Here's how the part is built. I have some questions about the finished solid (model axes, mm). Face numbers are marked on the shaded views. Coordinates: 2 decimals unless noted, no trailing zeros. Write each loop counter-clockwise with the first axis right and the second up, starting at its lowest first coordinate (ties: lowest second). Pieces come first, ordered by that corner, then holes. Notation, with made-up numbers: (-38, 2.25) - (0, 2.25) arc R16 cw to (0, 20.25) - close; hole circle Ø11 at (26, 71.5). An arc over 180 degrees is marked (long way). Answer in a Markdown table with one row per item. Add a question column.
Item 1: Imagine slicing it at A-A (x = 127). Please give me the cut outline in (y, z), plus the area to 3 significant figures.
Item 2: If I drill on probe 1 along Z at (x, y) = (25.4, -17.5); probe 2 along X at (y, z) = (-17.25, -70); probe 3 along X at (y, z) = (-11, -94.5), over which ranges is the centre line in solid material (lowest first)? Write a range as from..to.
Item 3: Imagine slicing it at C-C (y = -21.5). State how many separate pieces and enclosed holes the cut face has, plus the area to 3 significant figures.
Item 4: Imagine slicing it at B-B (z = -63.5). Please give me the cut outline in (x, y).
Item 5: We'd pull the mould along X, two halves only. Please class the marked faces 1, 2, 3 and 4: +X half, -X half, draft (parallel to the pull), parting line (faces both ways), or undercut.
Item 6: Imagine slicing it at D-D (z = -97.5). Please give me the cut outline in (x, y).
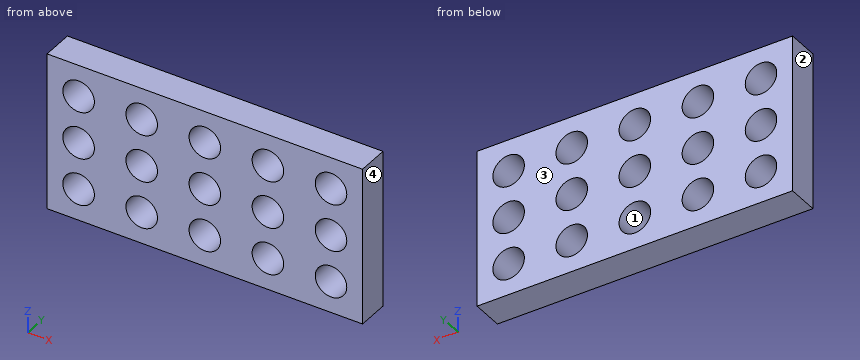
from build123d import *

# Parameters (mm, degrees)
F0_W     = 254
F0_H     = 127
F0_R     = 12.7
F1_DEPTH = 25.4


with BuildPart() as f1:
    # F0 (on Front) → F1 (new body)
    with BuildSketch(Plane.XZ):
        with Locations((127, -63.5)):
            Rectangle(F0_W, F0_H)
        with Locations((25.4, -101.6)):
            Circle(F0_R, mode=Mode.SUBTRACT)
        with Locations((76.2, -101.6)):
            Circle(F0_R, mode=Mode.SUBTRACT)
        with Locations((127, -101.6)):
            Circle(F0_R, mode=Mode.SUBTRACT)
        with Locations((177.8, -101.6)):
            Circle(F0_R, mode=Mode.SUBTRACT)
        with Locations((228.6, -101.6)):
            Circle(F0_R, mode=Mode.SUBTRACT)
        with Locations((25.4, -63.5)):
            Circle(F0_R, mode=Mode.SUBTRACT)
        with Locations((76.2, -63.5)):
            Circle(F0_R, mode=Mode.SUBTRACT)
        with Locations((25.4, -25.4)):
            Circle(F0_R, mode=Mode.SUBTRACT)
        with Locations((76.2, -25.4)):
            Circle(F0_R, mode=Mode.SUBTRACT)
        with Locations((127, -63.5)):
            Circle(F0_R, mode=Mode.SUBTRACT)
        with Locations((177.8, -63.5)):
            Circle(F0_R, mode=Mode.SUBTRACT)
        with Locations((228.6, -63.5)):
            Circle(F0_R, mode=Mode.SUBTRACT)
        with Locations((127, -25.4)):
            Circle(F0_R, mode=Mode.SUBTRACT)
        with Locations((177.8, -25.4)):
            Circle(F0_R, mode=Mode.SUBTRACT)
        with Locations((228.6, -25.4)):
            Circle(F0_R, mode=Mode.SUBTRACT)
    extrude(amount=F1_DEPTH)


solid = f1.part
Here are the results:
| question | item | result |
|---|---|---|
| 1 | outline | (-25.4, -127) - (0, -127) - (0, -114.3) - (-25.4, -114.3) - close; (-25.4, -88.9) - (0, -88.9) - (0, -76.2) - (-25.4, -76.2) - close; (-25.4, -50.8) - (0, -50.8) - (0, -38.1) - (-25.4, -38.1) - close; (-25.4, -12.7) - (0, -12.7) - (0, 0) - (-25.4, 0) - close |
| 1 | area | 1,290 mm2 |
| 2 | probe 1 | z = -127..-114.3, -88.9..-76.2, -50.8..-38.1, -12.7..0 |
| 2 | probe 2 | x = 0..14.49, 36.31..65.29, 87.11..116.09, 137.91..166.89, 188.71..217.69, 239.51..254 |
| 2 | probe 3 | x = 0..14.87, 35.93..65.67, 86.73..116.47, 137.53..167.27, 188.33..218.07, 239.13..254 |
| 3 | separate pieces | 1 |
| 3 | enclosed holes | 15 |
| 3 | area | 24,700 mm2 |
| 4 | outline | (0, -25.4) - (12.7, -25.4) - (12.7, 0) - (0, 0) - close; (38.1, -25.4) - (63.5, -25.4) - (63.5, 0) - (38.1, 0) - close; (88.9, -25.4) - (114.3, -25.4) - (114.3, 0) - (88.9, 0) - close; (139.7, -25.4) - (165.1, -25.4) - (165.1, 0) - (139.7, 0) - close; (190.5, -25.4) - (215.9, -25.4) - (215.9, 0) - (190.5, 0) - close; (241.3, -25.4) - (254, -25.4) - (254, 0) - (241.3, 0) - close |
| 5 | face 1 | undercut |
| 5 | face 2 | -X half |
| 5 | face 3 | draft |
| 5 | face 4 | +X half |
| 6 | outline | (0, -25.4) - (13.38, -25.4) - (13.38, 0) - (0, 0) - close; (37.42, -25.4) - (64.18, -25.4) - (64.18, 0) - (37.42, 0) - close; (88.22, -25.4) - (114.98, -25.4) - (114.98, 0) - (88.22, 0) - close; (139.02, -25.4) - (165.78, -25.4) - (165.78, 0) - (139.02, 0) - close; (189.82, -25.4) - (216.58, -25.4) - (216.58, 0) - (189.82, 0) - close; (240.62, -25.4) - (254, -25.4) - (254, 0) - (240.62, 0) - close |
